Answer from the drawing. Dimensions are ordinates in mm from the lowest x, y and z of the part. A direction names the side the tool comes from. Round coordinates to 2 decimals unless told otherwise and drop trailing zeros. Order: outer loops, then holes, each group sorted by start corner. A loop starts at its lowest first (then second) coordinate and runs counter-clockwise, first axis right, second up. Notation, with made-up numbers: (75.5, 87.25) -> (101.5, 87.25) arc R25 ccw to (101.5, 109.25) -> close; hole circle Ø4 at (-37, 40.5). An arc over 180 degrees is marked (long way). Use a Markdown table: item, result. Add a question column.
Item 1: Find the intervals of material crossed by L1, parallel to Y at x = 11, z = 1.2; L2, parallel to Y at x = 11, z = 3.75, in increasing order. Write a range as [from, to].
Item 2: A tool of negligible diameter and unlimited length cuts with its end or side. For the marked faces 1, 2 and 3, from which of +Z, -Z, +X, -X, +Y, -Y can it reach the whole face along a straight path? Write none if from no direction.
Item 3: A cutting plane is placed at C-C, the plane y = 19. Determine the outline of the cut face in (x, z), plus the area to 3 significant figures.
Item 4: Flat-ended cylindrical pins translate along their axes: P1, Ø1, axis at y = 19, z = 2, coming from the -X side; P2, Ø3, axis at y = 9.5, z = 6.5, coming from the -X side; P3, Ø1.8, axis at x = 11, y = 3, coming from the +Z side; P4, Ø2.5, axis at x = 11, z = 8, coming from the +Y side. Find the tip coordinate at first contact, or state that the pin passes through.
Item 5: A cutting plane is placed at B-B, the plane x = 9. Determine the outline of the cut face in (y, z).
Item 6: A cutting plane is placed at A-A, the plane y = 11. Determine the outline of the cut face in (x, z).
Item 7: For a pull along X with two mould halves and no side action, classify the marked faces 4, 5 and 6 as +X half, -X half, draft (parallel to the pull), parting line (faces both ways), or undercut.
Item 8: A cutting plane is placed at D-D, the plane x = 12. Determine the outline of the cut face in (y, z).
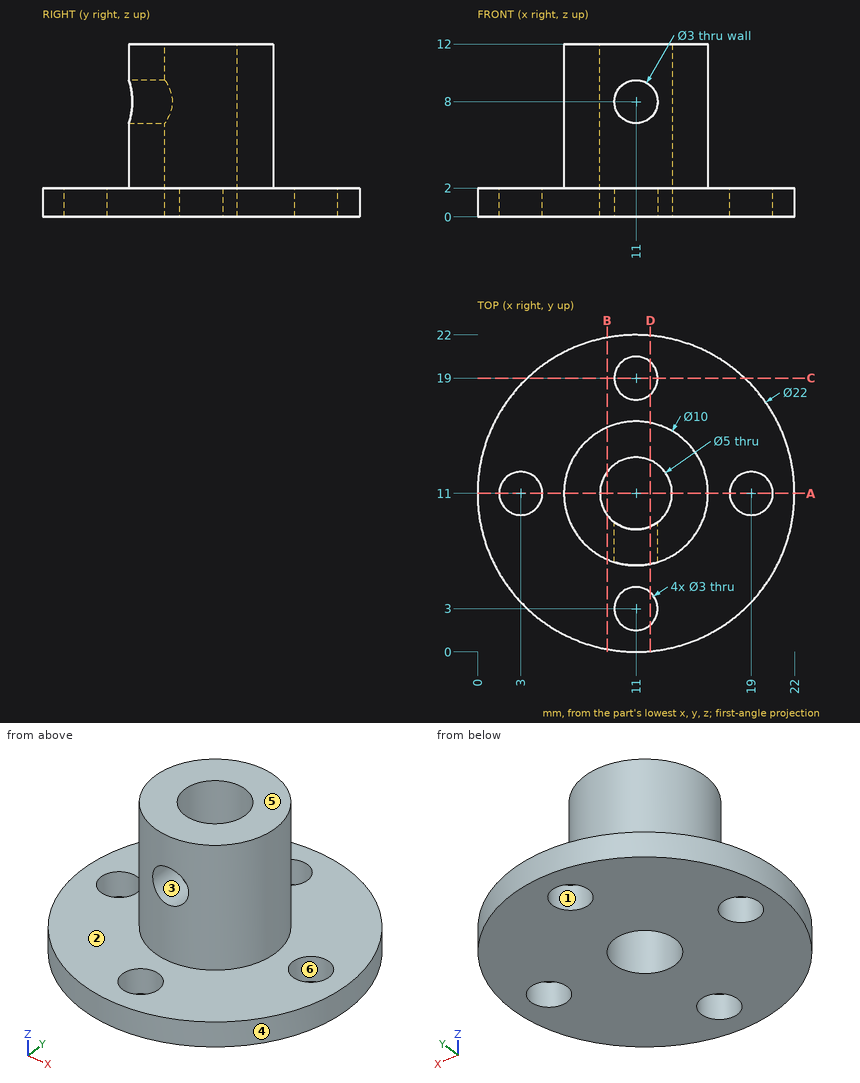
Reported:
| question | item | result |
|---|---|---|
| 1 | L1 | [0, 1.5], [4.5, 8.5], [13.5, 17.5], [20.5, 22] |
| 1 | L2 | [6, 8.5], [13.5, 16] |
| 2 | face 1 | +Z, -Z |
| 2 | face 2 | +Z |
| 2 | face 3 | -Y |
| 3 | outline | (3.45, 0) -> (9.5, 0) -> (9.5, 2) -> (3.45, 2) -> close; (12.5, 0) -> (18.55, 0) -> (18.55, 2) -> (12.5, 2) -> close |
| 3 | area | 24.2 mm² |
| 4 | P1 | x = 2.95 |
| 4 | P2 | x = 6 |
| 4 | P3 | through |
| 4 | P4 | y = 16 |
| 5 | outline | (0.18, 0) -> (9.5, 0) -> (9.5, 12) -> (6.42, 12) -> (6.42, 2) -> (0.18, 2) -> close; (12.5, 0) -> (21.82, 0) -> (21.82, 2) -> (15.58, 2) -> (15.58, 12) -> (12.5, 12) -> close |
| 6 | outline | (0, 0) -> (1.5, 0) -> (1.5, 2) -> (0, 2) -> close; (4.5, 0) -> (8.5, 0) -> (8.5, 12) -> (6, 12) -> (6, 2) -> (4.5, 2) -> close; (13.5, 0) -> (17.5, 0) -> (17.5, 2) -> (16, 2) -> (16, 12) -> (13.5, 12) -> close; (20.5, 0) -> (22, 0) -> (22, 2) -> (20.5, 2) -> close |
| 7 | face 4 | parting line |
| 7 | face 5 | draft |
| 7 | face 6 | undercut |
| 8 | outline | (0.05, 0) -> (1.88, 0) -> (1.88, 2) -> (0.05, 2) -> close; (4.12, 0) -> (8.71, 0) -> (8.71, 6.88) -> (6.1, 6.88) -> (6.1, 2) -> (4.12, 2) -> close; (6.1, 9.12) -> (8.71, 9.12) -> (8.71, 12) -> (6.1, 12) -> close; (13.29, 0) -> (17.88, 0) -> (17.88, 2) -> (15.9, 2) -> (15.9, 12) -> (13.29, 12) -> close; (20.12, 0) -> (21.95, 0) -> (21.95, 2) -> (20.12, 2) -> close |
